```python
from build123d import *

# Parameters (mm, degrees)
SKETCH1_W           = 17.78
SKETCH1_H           = 17.78
SKETCH1_R           = 2.0999958
BOSS_EXTRUDE1_DEPTH = 2.54
SKETCH2_R           = 1.016
BOSS_EXTRUDE2_DEPTH = 7.62


with BuildPart() as part:
    # Sketch1 → Boss-Extrude1 (new body)
    with BuildSketch(Plane.XY):
        with Locations((8.89, 8.89)):
            Rectangle(SKETCH1_W, SKETCH1_H)
        with Locations((8.89, 5.08)):
            Circle(SKETCH1_R, mode=Mode.SUBTRACT)
    extrude(amount=-BOSS_EXTRUDE1_DEPTH)

    # Sketch2 → Boss-Extrude2 (add)
    with BuildSketch(Plane(origin=(0, 17.78, 0), x_dir=(1, 0, 0), z_dir=(0, 1, 0))):
        with Locations(Location((2.54, 1.27, 0), (0, 0, 90))):
            Circle(SKETCH2_R)
        with Locations(Location((15.24, 1.27, 0), (0, 0, 90))):
            Circle(SKETCH2_R)
    extrude(amount=BOSS_EXTRUDE2_DEPTH)


solid = part.part
```
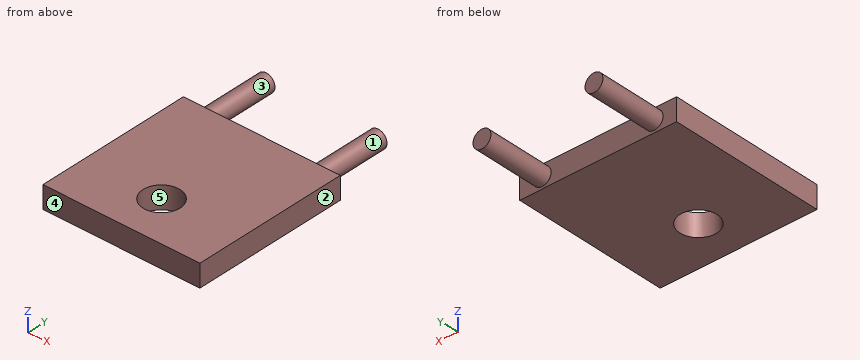
Build history of the part. All positions in model axes, mm. Face numbers are marked on the shaded views. A direction names the side the tool comes from. Round coordinates to 2 decimals unless told otherwise and drop trailing zeros. Loops run counter-clockwise (first coordinate to the right, second up) from the corner with the lowest first, then second, coordinate; pieces in that order, holes last.
Item 1: Drill centre lines: line 1 along Y through (x, z) = (9, -1.85); line 2 along Y through (x, z) = (13.75, -1.15); line 3 along X through (y, z) = (20.25, -1.8). Where is each one in solid material? Low to high.
Item 2: Saw through at C-C (x = 15.24). List the corners of the cut face in (y, z), then the cut area to 3 significant figures.
Item 3: Saw through at A-A (y = 5.08). List the corners of the cut face in (x, z), then the cut area to 3 significant figures.
Item 4: Saw through at D-D (x = 9.5). List the corners of the cut face in (y, z).
Item 5: Saw through at B-B (z = -1.27). List the corners of the cut face in (x, y), then the cut area to 3 significant figures.
Item 6: Which spindle directions (+Z, -Z, +X, -X, +Y, -Y) get a long thin tool onto all of the face, cutting with end or side? Do the marked faces 1 and 2. Say none if no direction does.
Item 7: Pin check, flat tips, straight feed: P1, Ø8, axis at x = 3.5, y = 13.5, coming from the +Z side; P2, Ø1.5, axis at y = 21.5, z = -0.5, coming from the +X side. Stop position of each tip, or through.
Item 8: Two-plate mould, pull along Y, no slides. Class the marked faces 3, 4 and 5: released by +Y, released by -Y, zero draft, split by the parting line, or undercut.
Worked answers:
1. line 1: y = 0 to 2.98, 7.18 to 17.78
1. line 2: y = 0 to 17.78
1. line 3: x = 1.67 to 3.41, 14.37 to 16.11
2. outline: (0, -2.54) - (17.78, -2.54) - (17.78, -2.29) - (25.4, -2.29) - (25.4, -0.25) - (17.78, -0.25) - (17.78, 0) - (0, 0) - close
2. area: 60.6 mm2
3. outline: (0, -2.54) - (6.79, -2.54) - (6.79, 0) - (0, 0) - close; (10.99, -2.54) - (17.78, -2.54) - (17.78, 0) - (10.99, 0) - close
3. area: 34.5 mm2
4. outline: (0, -2.54) - (3.07, -2.54) - (3.07, 0) - (0, 0) - close; (7.09, -2.54) - (17.78, -2.54) - (17.78, 0) - (7.09, 0) - close
5. outline: (0, 0) - (17.78, 0) - (17.78, 17.78) - (16.26, 17.78) - (16.26, 25.4) - (14.22, 25.4) - (14.22, 17.78) - (3.56, 17.78) - (3.56, 25.4) - (1.52, 25.4) - (1.52, 17.78) - (0, 17.78) - close; hole circle Ø4.2 at (8.89, 5.08)
5. area: 333 mm2
6. face 1: +Y
6. face 2: +Z, -Z, +X, +Y, -Y
7. P1: stops at z = 0
7. P2: stops at x = 16.26
8. face 3: zero draft
8. face 4: released by -Y
8. face 5: undercut
